Work out the finished part from the listing and answer in its coordinate system (mm). Round coordinates to 2 decimals unless told otherwise and drop trailing zeros. Order: outer loops, then holes, each group sorted by start corner. A loop starts at its lowest first (then second) coordinate and runs counter-clockwise, first axis right, second up. Notation, with made-up numbers: M 38,-33.5 L 96,-33.5 A18 cw 96,-19.5 Z; hole C 30,-11.75 d9. An arc over 180 degrees is marked long. Answer as a JSON object with one key per item and string values. Group by question number.
from build123d import *

# Parameters (mm, degrees)
CROQUIS1_W              = 80
CROQUIS1_H              = 20
CROQUIS1_R              = 2
CROQUIS1_R_2            = 4.05
SALIENTE_EXTRUIR2_DEPTH = 5
CROQUIS2_R              = 6
SALIENTE_EXTRUIR3_DEPTH = 2.1


with BuildPart() as part:
    # Croquis1 → Saliente-Extruir2 (new body)
    with BuildSketch(Plane.XY):
        with Locations((40, 10)):
            Rectangle(CROQUIS1_W, CROQUIS1_H)
        with Locations((30, 10)):
            Circle(CROQUIS1_R, mode=Mode.SUBTRACT)
        with Locations((50, 10)):
            Circle(CROQUIS1_R, mode=Mode.SUBTRACT)
        with Locations((8, 10)):
            Circle(CROQUIS1_R_2, mode=Mode.SUBTRACT)
        with Locations((72, 10)):
            Circle(CROQUIS1_R_2, mode=Mode.SUBTRACT)
    extrude(amount=SALIENTE_EXTRUIR2_DEPTH)

    # Croquis2 → Saliente-Extruir3 (add)
    with BuildSketch(Plane.XY.offset(5)):
        with Locations((8, 10)):
            Circle(CROQUIS2_R)
        with Locations((73, 10)):
            Circle(CROQUIS2_R)
    extrude(amount=-SALIENTE_EXTRUIR3_DEPTH)


solid = part.part
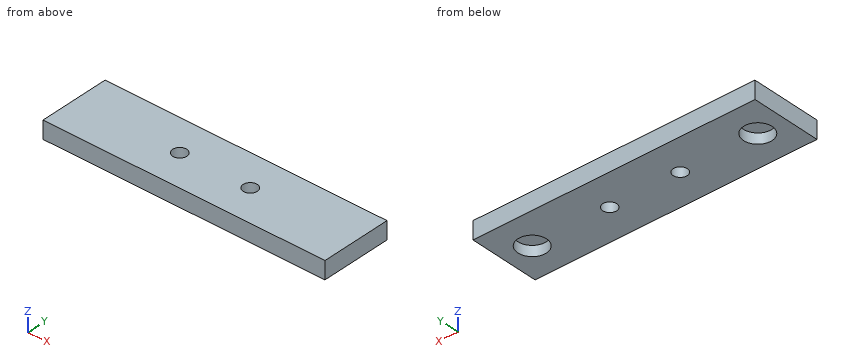
Item 1: Each of these flat-tipped pins is pushed along its axis until it touches: pin 1 (5 mm diameter, centred on x = 72, y = 10, fed in from -Z); pin 2 (3.5 mm diameter, centred on x = 50, y = 10, fed in from +Z). Where does it stop, or does it pass through?
Item 2: Consider L1, parallel to Y at x = 30, z = 2.85; L2, parallel to Y at x = 8, z = 1.25; L3, parallel to Z at x = 10.5, y = 13. Determine where each line is inside the solid, lowest interval first.
Item 3: Find section A-A (y = 10). Give the vertices of the cut face in (x, z), and give its area (3 significant figures).
Item 4: Find section B-B (x = 30). Give the vertices of the cut face in (y, z).
Item 5: Find section C-C (z = 2.05). Give the vertices of the cut face in (x, y), and give its area (3 significant figures).
Item 6: Find section D-D (x = 72). Give the vertices of the cut face in (y, z).
Responses:
{
 "1": {"pin 1": "stops at z = 2.9", "pin 2": "passes through"},
 "2": {"L1": "y = 0 to 8, 12 to 20", "L2": "y = 0 to 5.95, 14.05 to 20", "L3": "z = 2.9 to 5"},
 "3": {"outline": "M 0,0 L 3.95,0 L 3.95,2.9 L 12.05,2.9 L 12.05,0 L 28,0 L 28,5 L 0,5 Z; M 32,0 L 48,0 L 48,5 L 32,5 Z; M 52,0 L 67.95,0 L 67.95,2.9 L 76.05,2.9 L 76.05,0 L 80,0 L 80,5 L 52,5 Z", "area": "313 mm^2"},
 "4": {"outline": "M 0,0 L 8,0 L 8,5 L 0,5 Z; M 12,0 L 20,0 L 20,5 L 12,5 Z"},
 "5": {"outline": "M 0,0 L 80,0 L 80,20 L 0,20 Z; hole C 8,10 d8.1; hole C 30,10 d4; hole C 50,10 d4; hole C 72,10 d8.1", "area": "1,470 mm^2"},
 "6": {"outline": "M 0,0 L 5.95,0 L 5.95,2.9 L 14.05,2.9 L 14.05,0 L 20,0 L 20,5 L 0,5 Z"}
}
